Part model, mm, in its own coordinate system. A direction names the side the tool comes from. Round coordinates to 2 decimals unless told otherwise and drop trailing zeros. Loops run counter-clockwise (first coordinate to the right, second up) from the corner with the lowest first, then second, coordinate; pieces in that order, holes last. Notation, with made-up numbers: (8.5, -35) -> (31.5, -35) arc R11 ccw to (31.5, -14) -> close; hole circle Ø2 at (-11.5, 71.5). An arc over 180 degrees is marked (long way). Answer as a JSON object with one key per item and string values. Group by question number.
from build123d import *

# Parameters (mm, degrees)
F0_W     = 24
F0_H     = 24
F1_DEPTH = 58
F2_R     = 1.85
F3_DEPTH = 7.5


with BuildPart() as f1:
    # F0 (on Top) → F1 (new body)
    with BuildSketch(Plane.XY):
        Rectangle(F0_W, F0_H)
        with BuildLine():
            ThreePointArc((-8.7, -10.2), (-9.76066, -9.76066), (-10.2, -8.7))
            Line((-10.2, -8.7), (-10.2, -3))
            Line((-10.2, -3), (-6.2, -3))
            ThreePointArc((-6.2, -3), (-5.492893, -2.707107), (-5.2, -2))
            Line((-5.2, -2), (-5.2, 2))
            ThreePointArc((-5.2, 2), (-5.492893, 2.707107), (-6.2, 3))
            Line((-6.2, 3), (-10.2, 3))
            Line((-10.2, 3), (-10.2, 8.7))
            ThreePointArc((-10.2, 8.7), (-9.76066, 9.76066), (-8.7, 10.2))
            Line((-8.7, 10.2), (-3, 10.2))
            Line((-3, 10.2), (-3, 6.2))
            ThreePointArc((-3, 6.2), (-2.707107, 5.492893), (-2, 5.2))
            Line((-2, 5.2), (2, 5.2))
            ThreePointArc((2, 5.2), (2.707107, 5.492893), (3, 6.2))
            Line((3, 6.2), (3, 10.2))
            Line((3, 10.2), (8.7, 10.2))
            ThreePointArc((8.7, 10.2), (9.76066, 9.76066), (10.2, 8.7))
            Line((10.2, 8.7), (10.2, 3))
            Line((10.2, 3), (6.2, 3))
            ThreePointArc((6.2, 3), (5.492893, 2.707107), (5.2, 2))
            Line((5.2, 2), (5.2, -2))
            ThreePointArc((5.2, -2), (5.492893, -2.707107), (6.2, -3))
            Line((6.2, -3), (10.2, -3))
            Line((10.2, -3), (10.2, -8.7))
            ThreePointArc((10.2, -8.7), (9.76066, -9.76066), (8.7, -10.2))
            Line((8.7, -10.2), (3, -10.2))
            Line((3, -10.2), (3, -6.2))
            ThreePointArc((3, -6.2), (2.707107, -5.492893), (2, -5.2))
            Line((2, -5.2), (-2, -5.2))
            ThreePointArc((-2, -5.2), (-2.707107, -5.492893), (-3, -6.2))
            Line((-3, -6.2), (-3, -10.2))
            Line((-3, -10.2), (-8.7, -10.2))
        make_face(mode=Mode.SUBTRACT)
    extrude(amount=F1_DEPTH)

    # F2 (on face) → F3 (cut)
    with BuildSketch(Plane.XZ.offset(12)):
        with Locations((0, 53)):
            Circle(F2_R)
        with Locations((8, 45)):
            Circle(F2_R)
        with Locations((-8, 45)):
            Circle(F2_R)
        with Locations((0, 37)):
            Circle(F2_R)
        with Locations((-8, 29)):
            Circle(F2_R)
        with Locations((0, 21)):
            Circle(F2_R)
        with Locations((8, 29)):
            Circle(F2_R)
        with Locations((8, 13)):
            Circle(F2_R)
        with Locations((-8, 13)):
            Circle(F2_R)
        with Locations((0, 5)):
            Circle(F2_R)
    extrude(amount=-F3_DEPTH, mode=Mode.SUBTRACT)


solid = f1.part
Item 1: Two-plate mould, pull along Z, no slides. Class faces 4 (the face through (9.765, -11.108, 45.556)), 5 (the face through (0, 6, 58)), 6 (the face through (-12, 0, 29)): pulls with the +Z half, pulls with the -Z half, needs draft (parallel to the pull), parting line crosses it, or undercut.
Item 2: Band-saw the part on C-C, the plane x = 7.25. List the corners of the cut face in (y, z), plus the area to 3 significant figures.
Item 3: Band-saw the part on B-B, the plane y = -4.5. List the corners of the cut face in (x, z), plus the area to 3 significant figures.
Item 4: Drill centre lines: line 1 (Z direction, x = 0, y = -10.25); line 2 (X direction, y = 7, z = 7); line 3 (X direction, y = -10.15, z = 13). Where is each one in solid material? Low to high.
Item 5: Band-saw the part on A-A, the plane x = 0. List the corners of the cut face in (y, z).
Item 6: Which spindle directions (+Z, -Z, +X, -X, +Y, -Y) get a long thin tool onto all of the face, cutting with end or side? Do faces 1 (the face through (6, -10.2, 29)), 2 (the face through (-9.85, -11.11, 29.08)), 3 (the face through (0, 12, 29)). Say none if no direction does.
Entries:
{
 "1": {"face 4": "undercut", "face 5": "pulls with the +Z half", "face 6": "needs draft"},
 "2": {"outline": "(-12, 0) -> (-10.2, 0) -> (-10.2, 11.31) -> (-12, 11.31) -> close; (-12, 14.69) -> (-10.2, 14.69) -> (-10.2, 27.31) -> (-12, 27.31) -> close; (-12, 30.69) -> (-10.2, 30.69) -> (-10.2, 43.31) -> (-12, 43.31) -> close; (-12, 46.69) -> (-10.2, 46.69) -> (-10.2, 58) -> (-12, 58) -> close; (-3, 0) -> (3, 0) -> (3, 58) -> (-3, 58) -> close; (10.2, 0) -> (12, 0) -> (12, 58) -> (10.2, 58) -> close", "area": "539 mm²"},
 "3": {"outline": "(-12, 0) -> (-10.2, 0) -> (-10.2, 58) -> (-12, 58) -> close; (10.2, 0) -> (12, 0) -> (12, 58) -> (10.2, 58) -> close", "area": "209 mm²"},
 "4": {"line 1": "0 to 3.15, 6.85 to 19.15, 22.85 to 35.15, 38.85 to 51.15, 54.85 to 58", "line 2": "-12 to -10.2, -3 to 3, 10.2 to 12", "line 3": "-12 to -9.85, -3 to 3, 9.85 to 12"},
 "5": {"outline": "(-12, 0) -> (-5.2, 0) -> (-5.2, 3.15) -> (-12, 3.15) -> close; (-12, 6.85) -> (-5.2, 6.85) -> (-5.2, 19.15) -> (-12, 19.15) -> close; (-12, 22.85) -> (-5.2, 22.85) -> (-5.2, 35.15) -> (-12, 35.15) -> close; (-12, 38.85) -> (-5.2, 38.85) -> (-5.2, 51.15) -> (-12, 51.15) -> close; (-12, 54.85) -> (-5.2, 54.85) -> (-5.2, 58) -> (-12, 58) -> close; (5.2, 0) -> (12, 0) -> (12, 58) -> (5.2, 58) -> close"},
 "6": {"face 1": "+Z, -Z", "face 2": "-Y", "face 3": "+Z, -Z, +X, -X, +Y"}
}
